Read the model definition and answer for the solid it produces. Units are mm, in the model's axes. A direction names the side the tool comes from. Give positions to 0.01 mm unless a question says otherwise; leave off trailing zeros. Order: outer loops, then holes, each group sorted by start corner. A loop starts at its lowest first (then second) coordinate and runs counter-clockwise, first axis right, second up. Notation, with made-up numbers: (-16, -16) - (-4, -16) arc R22 ccw to (-4, 1) - close; hole circle Ø7 at (5.5, -6.5). An arc over 180 degrees is marked (long way). One line per item, written item: value. Start each with the question number.
```python
from build123d import *

# Parameters (mm, degrees)
ESQUISSE1_R             = 20.32
ESQUISSE1_R_2           = 3.175
BOSS_EXTRU_1_DEPTH      = 5.08
ESQUISSE2_R             = 3.175
BOSS_EXTRU_2_DEPTH      = 28.575
ENL_V_MAT_EXTRU_1_DEPTH = 23.495
ESQUISSE4_R             = 4.097809842
BOSS_EXTRU_3_DEPTH      = 5.08
ESQUISSE5_R             = 9.525
ESQUISSE5_R_2           = 3.175
BOSS_EXTRU_4_DEPTH      = 6.35
CONG_1_R                = 3.175


with BuildPart() as part:
    # Esquisse1 → Boss.-Extru.1 (new body)
    with BuildSketch(Plane.XY):
        Circle(ESQUISSE1_R)
        with Locations((9.525, 0)):
            Circle(ESQUISSE1_R_2, mode=Mode.SUBTRACT)
        Circle(ESQUISSE1_R_2, mode=Mode.SUBTRACT)
    extrude(amount=BOSS_EXTRU_1_DEPTH)

    # Esquisse2 → Boss.-Extru.2 (add)
    with BuildSketch(Plane.XY):
        with Locations((9.525, 0)):
            Circle(ESQUISSE2_R)
    extrude(amount=BOSS_EXTRU_2_DEPTH)

    # Esquisse3 → Enlèv. mat.-Extru.1 (cut)
    with BuildSketch(Plane.XY.offset(28.575)):
        Polygon((10.863482677, -81.610355532), (6.858308609, -1.723189492), (6.699328429, 1.447827743), (2.694154361, 81.334993784), (-157.08017772, 73.324645646), (-148.910849404, -89.620703669), align=None)
    extrude(amount=-ENL_V_MAT_EXTRU_1_DEPTH, mode=Mode.SUBTRACT)

    # Esquisse4 → Boss.-Extru.3 (add)
    with BuildSketch(Plane.XY.offset(5.08)):
        Circle(ESQUISSE4_R)
    extrude(amount=-BOSS_EXTRU_3_DEPTH)

    # Esquisse5 → Boss.-Extru.4 (add)
    with BuildSketch(Plane(origin=(0, 0, 0), x_dir=(-1, 0, 0), z_dir=(0, 0, -1))):
        Circle(ESQUISSE5_R)
        Circle(ESQUISSE5_R_2, mode=Mode.SUBTRACT)
    extrude(amount=BOSS_EXTRU_4_DEPTH)

    # Congé1
    cong_1_edges = [part.edges().sort_by_distance(p)[0] for p in [
        (12.696017235, 0.15898018, 5.08),
        (6.778818519, -0.137680874, 5.08),
        (9.525, 0, 0),
    ]]
    fillet(cong_1_edges, radius=CONG_1_R)


solid = part.part
```
1) Each of these flat-tipped pins is pushed along its axis until it touches: pin 1 (4 mm diameter, centred on y = 12, z = 1.5, fed in from +X); pin 2 (6 mm diameter, centred on x = -8, y = 12.5, fed in from -Z); pin 3 (1.5 mm diameter, centred on x = -1.5, z = 1, fed in from -Y). Where does it stop, or does it pass through?
2) Section D-D on x = -16 is taken. Write down the section's boundary in (y, z), plus the area to 3 significant figures.
3) The mould has two halves that part along Y. Classify faces 6 (the cylindrical face through (0.69, -3.1, -3.13)), 7 (the flat face through (0, 0, 5.08)), 8 (the cylindrical face through (-2.645, 20.147, 2.504)): +Y half, -Y half, draft (parallel to the pull), parting line (faces both ways), or undercut.
4) Section C-C on z = 18 is taken. Write down the section's boundary in (x, y) (3 decimals).
5) Section A-A on x = 0 is taken. Write down the section's boundary in (y, z) (3 decimals), plus the area to 3 significant figures.
6) For faces 1 (the flat face through (10, 0, 28.575)), 2 (the flat face through (-4, 0, -6.35)), 3 (the cylindrical face through (7.559, -5.796, -4.74)), 4 (the cylindrical face through (12.7, 0, 18.3)), 5 (the flat face through (6.78, -0.16, 18.56)), determine the directions among +Z, -Z, +X, -X, +Y, -Y from which every point of the face is accessible in a straight line to the end or side of a thin tool.
7) Section B-B on z = -1 is taken. Write down the section's boundary in (x, y) (3 decimals).
8) Find the intervals of material crossed by probe 1 along Y at (x, z) = (0, -3.5) (3 decimals); probe 2 along Z at (x, y) = (17.5, 7); probe 3 along Y at (x, z) = (0, -2) (3 decimals), in increasing order. Write a range as from..to.
Solved:
1. pin 1: stops at x = 17.69
1. pin 2: stops at z = -0.12
1. pin 3: stops at y = -20.31
2. outline: (-12.53, 0) - (12.53, 0) - (12.53, 5.08) - (-12.53, 5.08) - close
2. area: 127 mm2
3. face 6: undercut
3. face 7: draft
3. face 8: parting line
4. outline: (6.699, 1.448) - (6.858, -1.723) arc R3.175 ccw (long way) to start
5. outline: (-20.32, 0) - (-12.7, 0) arc R3.175 cw to (-9.525, -3.175) - (-9.525, -6.35) - (-3.175, -6.35) - (-3.175, 0) - (3.175, 0) - (3.175, -6.35) - (9.525, -6.35) - (9.525, -3.175) arc R3.175 cw to (12.7, 0) - (20.32, 0) - (20.32, 5.08) - (-20.32, 5.08) - close
5. area: 291 mm2
6. face 1: +Z, +X, -X, +Y, -Y
6. face 2: -Z, +X, -X, +Y, -Y
6. face 3: -Z
6. face 4: +Z
6. face 5: +Z, -X, -Y
7. outline: circle Ø20.774 at (0, 0); hole circle Ø6.35 at (0, 0)
8. probe 1: y = -9.525..-3.175, 3.175..9.525
8. probe 2: z = 0..5.08
8. probe 3: y = -9.75..-3.175, 3.175..9.75
